from build123d import *

# Parameters (mm, degrees)
BOSS_EXTRUDE1_START     = -163.416678
SKETCH1_R               = 7.9375
SKETCH1_R_2             = 6.4643
BOSS_EXTRUDE1_DEPTH     = 333.562160318
CUT_EXTRUDE1_DEPTH      = 171.515374573
CUT_EXTRUDE1_DEPTH_BACK = 171.515374573


with BuildPart() as part:
    # Sketch1 → Boss-Extrude1 (new body)
    with BuildSketch(Plane(origin=(0, 0, 0), x_dir=(1, 0, 0), z_dir=(0, 1, 0)).offset(BOSS_EXTRUDE1_START)):
        with Locations(Location((0, 0, 0), (0, 0, 270))):
            Circle(SKETCH1_R)
        with Locations(Location((0, 0, 0), (0, 0, 270))):
            Circle(SKETCH1_R_2, mode=Mode.SUBTRACT)
    extrude(amount=BOSS_EXTRUDE1_DEPTH)

    # Sketch2 → Cut-Extrude1 (cut, two sides: drawn at the far end of the back side and taken through both)
    with BuildSketch(Plane.XY.offset(-CUT_EXTRUDE1_DEPTH_BACK)):
        with BuildLine():
            Line((-3.175, 170.145482762), (3.175, 170.145482762))
            Line((3.175, 170.145482762), (3.175, 144.745482762))
            ThreePointArc((3.175, 144.745482762), (2.710032015, 143.622950747), (1.5875, 143.157982762))
            Line((1.5875, 143.157982762), (-1.5875, 143.157982762))
            ThreePointArc((-1.5875, 143.157982762), (-2.710032015, 143.622950747), (-3.175, 144.745482762))
            Line((-3.175, 144.745482762), (-3.175, 170.145482762))
        make_face()
    extrude(amount=CUT_EXTRUDE1_DEPTH + CUT_EXTRUDE1_DEPTH_BACK, mode=Mode.SUBTRACT)


solid = part.part
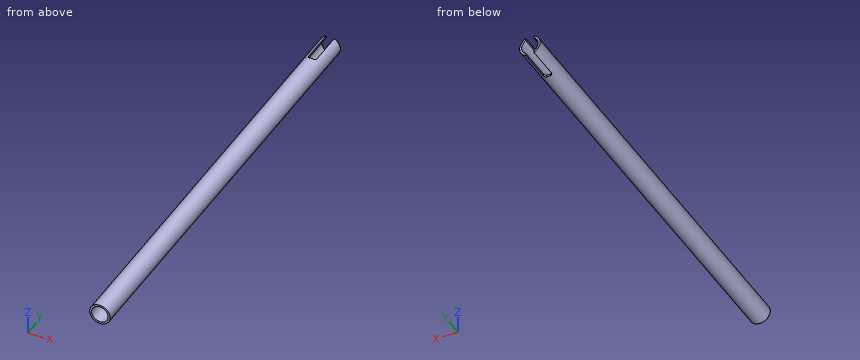
Geometry check sheet. Reference: the model listing, model coordinates, mm. Round coordinates to 2 decimals unless told otherwise and drop trailing zeros. Loops run counter-clockwise (first coordinate to the right, second up) from the corner with the lowest first, then second, coordinate; pieces in that order, holes last.
Item 1: Thickness scan on line 1 (Z direction, x = 1.5, y = 67); line 2 (Z direction, x = 0, y = -81.5). Record the ranges inside material, lowest first.
Item 2: Cross-section at A-A on z = 0. Record the boundary of the cut face in (x, y), then the cut area to 3 significant figures.
Item 3: Gauge pin test, flat ends, axial feed: pin 1 (0.8 mm diameter, centred on x = -0.5, z = -7, fed in from +Y); pin 2 (1.5 mm diameter, centred on x = 4, z = 0.5, fed in from -Y); pin 3 (1.8 mm diameter, centred on y = 160.5, z = -6, fed in from +X); pin 4 (2 mm diameter, centred on x = -1.5, y = 103.5, fed in from +Z). Record the tip position at first contact, or that the pin passes through.
Item 4: Cross-section at B-B on y = -21. Record the boundary of the cut face in (x, z) (1 decimal), then the cut area to 3 significant figures.
Answer sheet:
1. line 1: z = -7.79 to -6.29, 6.29 to 7.79
1. line 2: z = -7.94 to -6.46, 6.46 to 7.94
2. outline: (-7.94, -163.42) - (-6.46, -163.42) - (-6.46, 170.15) - (-7.94, 170.15) - close; (6.46, -163.42) - (7.94, -163.42) - (7.94, 170.15) - (6.46, 170.15) - close
2. area: 983 mm2
3. pin 1: stops at y = 143.16
3. pin 2: passes through
3. pin 3: stops at x = 6.08
3. pin 4: stops at z = 7.92
4. outline: circle Ø15.9 at (0, 0); hole circle Ø12.9 at (0, 0)
4. area: 66.7 mm2
